from build123d import *

# Parameters (mm, degrees)
F0_W     = 118
F0_H     = 118
F1_DEPTH = 52
F2_W     = 115.5
F2_H     = 115.5
F3_DEPTH = 51.3
F4_R     = 2
F5_DEPTH = 25


with BuildPart() as f1:
    # F0 (on Top) → F1 (new body)
    with BuildSketch(Plane.XY):
        Rectangle(F0_W, F0_H)
    extrude(amount=F1_DEPTH)

    # F2 (on face) → F3 (cut)
    with BuildSketch(Plane.XY.offset(52)):
        Rectangle(F2_W, F2_H)
    extrude(amount=-F3_DEPTH, mode=Mode.SUBTRACT)

    # F4 (on face) → F5 (cut)
    with BuildSketch(Plane(origin=(0, 0, 0), x_dir=(1, 0, 0), z_dir=(0, 0, -1))):
        with BuildLine():
            ThreePointArc((38.543689, 9.640613), (40.359387, 8.543689), (41.456311, 10.359387))
            ThreePointArc((41.456311, 10.359387), (0, 42.82883), (-41.456311, 10.359387))
            ThreePointArc((-41.456311, 10.359387), (-40.359387, 8.543689), (-38.543689, 9.640613))
            ThreePointArc((-38.543689, 9.640613), (0, 39.82883), (38.543689, 9.640613))
        make_face()
        with BuildLine():
            ThreePointArc((41.456311, -10.359387), (40.359387, -8.543689), (38.543689, -9.640613))
            ThreePointArc((38.543689, -9.640613), (0, -39.82883), (-38.543689, -9.640613))
            ThreePointArc((-38.543689, -9.640613), (-40.359387, -8.543689), (-41.456311, -10.359387))
            ThreePointArc((-41.456311, -10.359387), (0, -42.82883), (41.456311, -10.359387))
        make_face()
        with BuildLine():
            ThreePointArc((9.337938, -18.654015), (8.654015, -20.662062), (10.662062, -21.345985))
            ThreePointArc((10.662062, -21.345985), (23.950936, 0), (10.662062, 21.345985))
            ThreePointArc((10.662062, 21.345985), (8.654015, 20.662062), (9.337938, 18.654015))
            ThreePointArc((9.337938, 18.654015), (20.950936, 0), (9.337938, -18.654015))
        make_face()
        with BuildLine():
            ThreePointArc((-9.337938, -18.654015), (-20.950936, 0), (-9.337938, 18.654015))
            ThreePointArc((-9.337938, 18.654015), (-8.654015, 20.662062), (-10.662062, 21.345985))
            ThreePointArc((-10.662062, 21.345985), (-23.950936, 0), (-10.662062, -21.345985))
            ThreePointArc((-10.662062, -21.345985), (-8.654015, -20.662062), (-9.337938, -18.654015))
        make_face()
        Circle(F4_R)
    extrude(amount=-F5_DEPTH, mode=Mode.SUBTRACT)


solid = f1.part
Source: CAD feature listing. Evaluate the final solid. Frame: model axes, mm. A direction names the side the tool comes from. Round coordinates to 2 decimals unless told otherwise and drop trailing zeros. Loops run counter-clockwise (first coordinate to the right, second up) from the corner with the lowest first, then second, coordinate; pieces in that order, holes last. Notation, with made-up numbers: M 88.5,11 L 105.5,11 A21 cw 105.5,31 Z; hole C -14.75,61 d7. An arc over 180 degrees is marked long. Answer as CSV lines item,"result".
Q1. Pull-direction query (Y, two-part tool) for faces 1 (the face through (23.95, 0.37, 0.35)), 2 (the face through (59, -1, 26)), 3 (the face through (-1, -59, 26)); classes: +Y half, -Y half, draft (parallel to the pull), parting line (faces both ways), or undercut.
Verdict:
face 1,"undercut"
face 2,"draft"
face 3,"-Y half"
Q2. Line query: line 1 along Y through (x, z) = (0, 0.3); line 2 along X through (y, z) = (0, 0.4); line 3 along X through (y, z) = (-34, 49.5). Output: solid intervals per line, ascending.
Verdict:
line 1,"y = -59 to -42.83, -39.83 to -2, 2 to 39.83, 42.83 to 59"
line 2,"x = -59 to -23.95, -20.95 to -2, 2 to 20.95, 23.95 to 59"
line 3,"x = -59 to -57.75, 57.75 to 59"
Q3. Cut plane A-A (y = 0). Return the cut outline in (x, z), plus the area to 3 significant figures.
Verdict:
outline,"M -59,0 L -23.95,0 L -23.95,0.7 L -57.75,0.7 L -57.75,52 L -59,52 Z; M -20.95,0 L -2,0 L -2,0.7 L -20.95,0.7 Z; M 2,0 L 20.95,0 L 20.95,0.7 L 2,0.7 Z; M 23.95,0 L 59,0 L 59,52 L 57.75,52 L 57.75,0.7 L 23.95,0.7 Z"
area,"204 mm^2"
Q4. Cut plane D-D (z = 31.5). Return the cut outline in (x, y), plus the area to 3 significant figures.
Verdict:
outline,"M -59,-59 L 59,-59 L 59,59 L -59,59 Z; hole M -57.75,-57.75 L 57.75,-57.75 L 57.75,57.75 L -57.75,57.75 Z"
area,"584 mm^2"
Q5. Cut plane C-C (y = -50). Return the cut outline in (x, z).
Verdict:
outline,"M -59,0 L 59,0 L 59,52 L 57.75,52 L 57.75,0.7 L -57.75,0.7 L -57.75,52 L -59,52 Z"
Q6. Cut plane B-B (x = 40). Return the cut outline in (y, z), plus the area to 3 significant figures.
Verdict:
outline,"M -59,0 L -15.07,0 L -15.07,0.7 L -57.75,0.7 L -57.75,52 L -59,52 Z; M -8.5,0 L 8.5,0 L 8.5,0.7 L -8.5,0.7 Z; M 15.07,0 L 59,0 L 59,52 L 57.75,52 L 57.75,0.7 L 15.07,0.7 Z"
area,"202 mm^2"
Q7. Contact query for flat-ended pins moving along their axis: pin 1 (8 mm diameter, centred on x = -5, y = -47, fed in from -Z); pin 2 (5 mm diameter, centred on x = 0, y = 0, fed in from +Z). Output: stop coordinate, or through.
Verdict:
pin 1,"stops at z = 0"
pin 2,"stops at z = 0.7"
Q8. Reachability of faces 4 (the face through (-23.95, -0.37, 0.35)), 5 (the face through (12, 1, 0.7)), 6 (the face through (-1, 59, 26)) from +Z, -Z, +X, -X, +Y, -Y: full face, straight path, thin tool, end or side. Return the list, or none.
Verdict:
face 4,"+Z, -Z"
face 5,"+Z"
face 6,"+Z, -Z, +X, -X, +Y"
